```python
from build123d import *

# Parameters (mm, degrees)
F0_W     = 40
F0_H     = 50
F0_R     = 2.75
F1_DEPTH = 3
F2_SIZE  = 5
F3_W     = 15
F3_H     = 30
F4_DEPTH = 4
F6_DEPTH = 12.5


with BuildPart() as f1:
    # F0 (on Top) → F1 (new body)
    with BuildSketch(Plane.XY):
        Rectangle(F0_W, F0_H)
        with Locations((-10, -20)):
            Circle(F0_R, mode=Mode.SUBTRACT)
        with Locations((10, -20)):
            Circle(F0_R, mode=Mode.SUBTRACT)
        with Locations((-10, 20)):
            Circle(F0_R, mode=Mode.SUBTRACT)
        with Locations((10, 20)):
            Circle(F0_R, mode=Mode.SUBTRACT)
    extrude(amount=F1_DEPTH)

    # F2
    f2_edges = [f1.edges().sort_by_distance(p)[0] for p in [
        (-20, 25, 1.5),
        (20, 25, 1.5),
        (-20, -25, 1.5),
        (20, -25, 1.5),
    ]]
    chamfer(f2_edges, length=F2_SIZE)

    # F3 (on face) → F4 (join)
    with BuildSketch(Plane.XY.offset(3)):
        Rectangle(F3_W, F3_H)
    extrude(amount=F4_DEPTH)

    # F5 (on Right) → F6 (cut, symmetric)
    with BuildSketch(Plane.YZ):
        with BuildLine():
            ThreePointArc((7, 4), (9, 2), (11, 4))
            Line((11, 4), (7, 4))
        make_face()
        with BuildLine():
            Line((7, 4), (11, 4))
            ThreePointArc((11, 4), (9, 6), (7, 4))
        make_face()
        with BuildLine():
            ThreePointArc((-11, 4), (-9, 2), (-7, 4))
            Line((-7, 4), (-11, 4))
        make_face()
        with BuildLine():
            Line((-11, 4), (-7, 4))
            ThreePointArc((-7, 4), (-9, 6), (-11, 4))
        make_face()
        with BuildLine():
            ThreePointArc((-2, 4), (0, 2), (2, 4))
            Line((2, 4), (-2, 4))
        make_face()
        with BuildLine():
            Line((-2, 4), (2, 4))
            ThreePointArc((2, 4), (0, 6), (-2, 4))
        make_face()
    extrude(amount=F6_DEPTH, both=True, mode=Mode.SUBTRACT)


solid = f1.part
```
Can you work these out from the model? Positions are in its coordinate system, mm. A direction names the side the tool comes from. Coordinates: 2 decimals unless noted, no trailing zeros. Loops run counter-clockwise (first coordinate to the right, second up) from the corner with the lowest first, then second, coordinate; pieces in that order, holes last. Notation, with made-up numbers: (-17, 34) -> (-12, 34) arc R10 ccw to (-12, 38) -> close; hole circle Ø7 at (23.5, 80.25). An arc over 180 degrees is marked (long way). Answer as a JSON object with one key per item and string values.
1) Thinking about a two-plate mould opening in X: for faces 1 (the face through (18, -22, 1)), 2 (the face through (9.642, 22.727, 1.479)), 3 (the face through (-10.358, -17.273, 1.479)), 4 (the face through (-17, -23, 1)), which applies, pulls with the +X half, pulls with the -X half, needs draft (parallel to the pull), parting line crosses it, or undercut?
Results:
{"face 1": "pulls with the +X half", "face 2": "undercut", "face 3": "undercut", "face 4": "pulls with the -X half"}
2) For faces 5 (the face through (7.5, -0.2, 6.3)), 6 (the face through (-7.5, -0.2, 6.3)), 7 (the face through (12.5, 0, 2.6)), which set-ups out of +Z, -Z, +X, -X, +Y, -Y let a thin tool reach every point of the face, with its end or its side?
Results:
{"face 5": "+Z, +X, +Y, -Y", "face 6": "+Z, -X, +Y, -Y", "face 7": "+Z"}
3) Imagine slicing it at D-D (z = 1). Please give me the cut outline in (x, y).
Results:
{"outline": "(-20, -20) -> (-15, -25) -> (15, -25) -> (20, -20) -> (20, 20) -> (15, 25) -> (-15, 25) -> (-20, 20) -> close; hole circle Ø5.5 at (-10, -20); hole circle Ø5.5 at (-10, 20); hole circle Ø5.5 at (10, -20); hole circle Ø5.5 at (10, 20)"}
4) If I drill on line 1 (Y direction, x = -10, z = 1.5); line 2 (Y direction, x = -5.5, z = 4); line 3 (Y direction, x = 4.5, z = 5.75), over which ranges is the centre line in solid material (lowest first)?
Results:
{"line 1": "y = -25 to -22.75, -17.25 to 17.25, 22.75 to 25", "line 2": "y = -15 to -11, -7 to -2, 2 to 7, 11 to 15", "line 3": "y = -15 to -9.97, -8.03 to -0.97, 0.97 to 8.03, 9.97 to 15"}
5) Imagine slicing it at A-A (y = 0). Please give me the cut outline in (x, z).
Results:
{"outline": "(-20, 0) -> (20, 0) -> (20, 3) -> (12.5, 3) -> (12.5, 2) -> (-12.5, 2) -> (-12.5, 3) -> (-20, 3) -> close; (-7.5, 6) -> (7.5, 6) -> (7.5, 7) -> (-7.5, 7) -> close"}
6) Imagine slicing it at B-B (z = 4). Please give me the cut outline in (x, y), then the cut area to 3 significant figures.
Results:
{"outline": "(-7.5, -15) -> (7.5, -15) -> (7.5, -11) -> (-7.5, -11) -> close; (-7.5, -7) -> (7.5, -7) -> (7.5, -2) -> (-7.5, -2) -> close; (-7.5, 2) -> (7.5, 2) -> (7.5, 7) -> (-7.5, 7) -> close; (-7.5, 11) -> (7.5, 11) -> (7.5, 15) -> (-7.5, 15) -> close", "area": "270 mm^2"}
7) Imagine slicing it at C-C (x = 1.5). Please give me the cut outline in (y, z), then the cut area to 3 significant figures.
Results:
{"outline": "(-25, 0) -> (25, 0) -> (25, 3) -> (15, 3) -> (15, 7) -> (-15, 7) -> (-15, 3) -> (-25, 3) -> close; hole circle Ø4 at (-9, 4); hole circle Ø4 at (0, 4); hole circle Ø4 at (9, 4)", "area": "232 mm^2"}
8) For P1, Ø2, axis at y = -6.5, z = 5, coming from the +X side; P2, Ø9, axis at x = 10, y = 20, coming from the +Z side; P3, Ø1.2, axis at x = 1, z = 4.5, coming from the -Y side, each with a flat end and sliding along its axis, tell me the tip position at first contact or that it passes through.
Results:
{"P1": "stops at x = 7.5", "P2": "stops at z = 3", "P3": "stops at y = -15"}
